```python
from build123d import *

# Parameters (mm, degrees)
SKETCH_1_R          = 34
SKETCH_1_R_2        = 8
SKETCH_1_R_3        = 2.05
EXTRUDE_1_DEPTH     = 3
SKETCH_2_R          = 2.55
CUT_EXTRUDE_1_DEPTH = 10
CHAMFER_1_SIZE      = 2.1
CHAMFER_2_SIZE      = 2.6


with BuildPart() as part:
    # 草图1 → 凸台-拉伸1 (new body)
    with BuildSketch(Plane(origin=(0, 0, 0), x_dir=(1, 0, 0), z_dir=(0, 1, 0))):
        with Locations(Location((0, 0, 0), (0, 0, 270))):
            Circle(SKETCH_1_R)
        with Locations(Location((0, 0, 0), (0, 0, 270))):
            Circle(SKETCH_1_R_2, mode=Mode.SUBTRACT)
        with Locations(Location((9.899494937, 9.899494937, 0), (0, 0, 270))):
            Circle(SKETCH_1_R_3, mode=Mode.SUBTRACT)
        with Locations(Location((14, 0, 0), (0, 0, 270))):
            Circle(SKETCH_1_R_3, mode=Mode.SUBTRACT)
        with Locations(Location((9.899494937, -9.899494937, 0), (0, 0, 270))):
            Circle(SKETCH_1_R_3, mode=Mode.SUBTRACT)
        with Locations(Location((-9.899494937, -9.899494937, 0), (0, 0, 270))):
            Circle(SKETCH_1_R_3, mode=Mode.SUBTRACT)
        with Locations(Location((-14, 0, 0), (0, 0, 270))):
            Circle(SKETCH_1_R_3, mode=Mode.SUBTRACT)
        with Locations(Location((-9.899494937, 9.899494937, 0), (0, 0, 270))):
            Circle(SKETCH_1_R_3, mode=Mode.SUBTRACT)
    extrude(amount=EXTRUDE_1_DEPTH)

    # 草图2 → 切除-拉伸1 (cut)
    with BuildSketch(Plane(origin=(0, 0, 0), x_dir=(-1, 0, 0), z_dir=(0, -1, 0))):
        with Locations(Location((0, 18, 0), (0, 0, 90))):
            Circle(SKETCH_2_R)
        with Locations(Location((0, -18, 0), (0, 0, 90))):
            Circle(SKETCH_2_R)
    extrude(amount=-CUT_EXTRUDE_1_DEPTH, mode=Mode.SUBTRACT)

    # 倒角1
    chamfer_1_edges = [part.edges().sort_by_distance(p)[0] for p in [
        (-9.899494937, 0, 7.849494937),
        (9.899494937, 0, -11.949494937),
        (14, 0, -2.05),
        (9.899494937, 0, 7.849494937),
        (-9.899494937, 0, -11.949494937),
        (-14, 0, -2.05),
    ]]
    chamfer(chamfer_1_edges, length=CHAMFER_1_SIZE)

    # 倒角2
    chamfer_2_edges = [part.edges().sort_by_distance(p)[0] for p in [
        (0, 3, -15.45),
        (0, 3, 20.55),
    ]]
    chamfer(chamfer_2_edges, length=CHAMFER_2_SIZE)


solid = part.part
```
Build history of the part. All positions in model axes, mm. Round coordinates to 2 decimals unless told otherwise and drop trailing zeros. Loops run counter-clockwise (first coordinate to the right, second up) from the corner with the lowest first, then second, coordinate; pieces in that order, holes last.
Item 1: Saw through at D-D (x = 23). List the corners of the cut face in (y, z).
Item 2: Saw through at C-C (z = 18). List the corners of the cut face in (x, y).
Item 3: Pin check, flat tips, straight feed: P1, Ø1, axis at y = 1.5, z = -21.5, coming from the +X side; P2, Ø3.5, axis at x = -14, z = 0, coming from the +Y side; P3, Ø6.5, axis at x = 0, z = 18, coming from the +Y side. Stop position of each tip, or through.
Item 4: Drill centre lines: line 1 along X through (y, z) = (2.45, 0); line 2 along X through (y, z) = (0.2, 10.5); line 3 along X through (y, z) = (1.7, 10). Where is each one in solid material? Low to high.
Item 5: Saw through at B-B (z = 0). List the corners of the cut face in (x, y), then the cut area to 3 significant figures.
Item 6: Saw through at A-A (x = 0). List the corners of the cut face in (y, z), then the cut area to 3 significant figures.
Worked answers:
1. outline: (0, -25.04) - (3, -25.04) - (3, 25.04) - (0, 25.04) - close
2. outline: (-28.84, 0) - (-2.55, 0) - (-2.55, 0.4) - (-5.15, 3) - (-28.84, 3) - close; (2.55, 0) - (28.84, 0) - (28.84, 3) - (5.15, 3) - (2.55, 0.4) - close
3. P1: stops at x = 26.74
3. P2: passes through
3. P3: stops at y = 1.1
4. line 1: x = -34 to -16.05, -11.95 to -8, 8 to 11.95, 16.05 to 34
4. line 2: x = -32.34 to -13.8, -6 to 6, 13.8 to 32.34
4. line 3: x = -32.5 to -12.35, -7.45 to 7.45, 12.35 to 32.5
5. outline: (-34, 0) - (-18.15, 0) - (-16.05, 2.1) - (-16.05, 3) - (-34, 3) - close; (-11.95, 2.1) - (-9.85, 0) - (-8, 0) - (-8, 3) - (-11.95, 3) - close; (8, 0) - (9.85, 0) - (11.95, 2.1) - (11.95, 3) - (8, 3) - close; (16.05, 2.1) - (18.15, 0) - (34, 0) - (34, 3) - (16.05, 3) - close
5. area: 123 mm2
6. outline: (0, -34) - (3, -34) - (3, -23.15) - (0.4, -20.55) - (0, -20.55) - close; (0, -15.45) - (0.4, -15.45) - (3, -12.85) - (3, -8) - (0, -8) - close; (0, 8) - (3, 8) - (3, 12.85) - (0.4, 15.45) - (0, 15.45) - close; (0, 20.55) - (0.4, 20.55) - (3, 23.15) - (3, 34) - (0, 34) - close
6. area: 112 mm2
